Geometry: see drawing. Coordinates: mm, zero at the bounding-box minimum. A direction names the side the tool comes from. Coordinates: 2 decimals unless noted, no trailing zeros. Write each loop counter-clockwise with the first axis right and the second up, starting at its lowest first coordinate (ties: lowest second). Pieces come first, ordered by that corner, then holes. Notation, with made-up numbers: (-36.75, 87) -> (-9.75, 87) arc R15 ccw to (-9.75, 94) -> close; hole circle Ø9 at (10.5, 6.25). An arc over 180 degrees is marked (long way). Use one line per item in the form item = value. Start each with the question number.
(1) Ray query, line 1 along X through (y, z) = (216.25, 60); line 2 along Y through (x, z) = (129, 60); line 3 along Z through (x, y) = (120, 215). Return the intervals inside material, ascending.
(2) Cut plane C-C on y = 119.5. Return the cut outline in (x, z), plus the area to 3 significant figures.
(3) Cut plane A-A on z = 43. Return the cut outline in (x, y).
(4) First-contact query: pin 1 (1 mm diameter, centred on x = 136, z = 95, fed in from -Y); pin 2 (10.5 mm diameter, centred on y = 58.25, z = 60, fed in from +X); pin 3 (5 mm diameter, centred on x = 120, z = 20, fed in from +Y); pin 4 (2 mm diameter, centred on y = 30, z = 23.5, fed in from -X). Flat tips, straight axial feed; report the tip coordinate or a pass-through.
(5) Cut plane B-B on x = 45.5. Return the cut outline in (y, z), plus the area to 3 significant figures.
(6) Set-up query: the marked faces 1, 2 and 3. Return all of +Z, -Z, +X, -X, +Y, -Y with unobstructed straight access to the full face (end or side cutting, diameter ignored); none if empty.
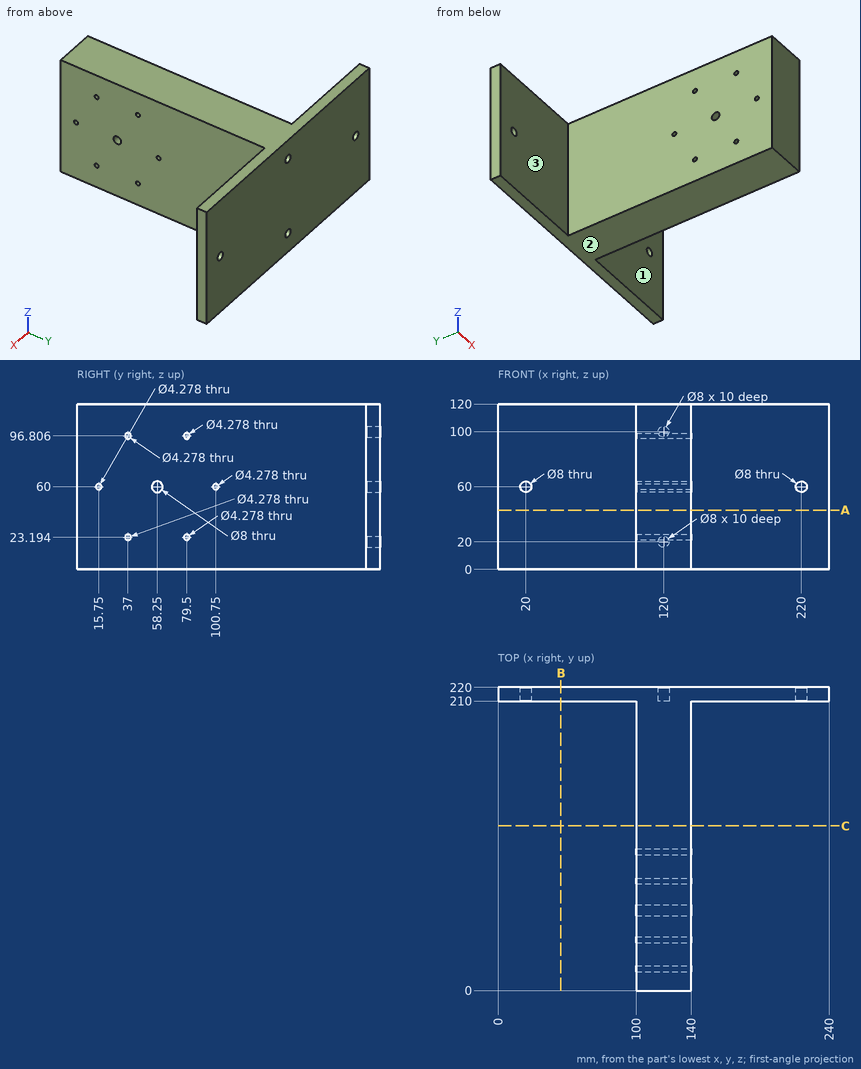
Values:
q1.line_1 = 0 to 16, 24 to 216, 224 to 240
q1.line_2 = 0 to 13.61, 17.89 to 54.25, 62.25 to 98.61, 102.89 to 220
q1.line_3 = 0 to 16, 24 to 96, 104 to 120
q2.outline = (100, 0) -> (140, 0) -> (140, 120) -> (100, 120) -> close
q2.area = 4,800 mm2
q3.outline = (0, 210) -> (100, 210) -> (100, 0) -> (140, 0) -> (140, 210) -> (240, 210) -> (240, 220) -> (0, 220) -> close
q4.pin_1 = 0
q4.pin_2 = 140
q4.pin_3 = 210
q4.pin_4 = 100
q5.outline = (210, 0) -> (220, 0) -> (220, 120) -> (210, 120) -> close
q5.area = 1,200 mm2
q6.face_1 = +Z, -Z, +X, -Y
q6.face_2 = -Z, +X, -X, +Y, -Y
q6.face_3 = +Z, -Z, -X, -Y
